```python
from build123d import *

# Parameters (mm, degrees)
CROQUIS1_R              = 4
CROQUIS1_R_2            = 1.25
SALIENTE_EXTRUIR1_DEPTH = 3.5
CROQUIS2_R              = 4
SALIENTE_EXTRUIR2_DEPTH = 150


with BuildPart() as part:
    # Croquis1 → Saliente-Extruir1 (new body)
    # profile 1 of 2: a face of its own
    with BuildSketch(Plane(origin=(0, 0, 0), x_dir=(1, 0, 0), z_dir=(0, 1, 0))):
        with BuildLine():
            Line((17.5, 2.5), (17.5, -2.5))
            ThreePointArc((17.5, -2.5), (16.035533906, -6.035533906), (12.5, -7.5))
            Line((12.5, -7.5), (-12.5, -7.5))
            ThreePointArc((-12.5, -7.5), (-16.035533906, -6.035533906), (-17.5, -2.5))
            Line((-17.5, -2.5), (-17.5, 2.5))
            ThreePointArc((-17.5, 2.5), (-16.035533906, 6.035533906), (-12.5, 7.5))
            Line((-12.5, 7.5), (12.5, 7.5))
            ThreePointArc((12.5, 7.5), (16.035533906, 6.035533906), (17.5, 2.5))
        make_face()
        Circle(CROQUIS1_R, mode=Mode.SUBTRACT)
        with Locations(Location((-13, 0, 0), (0, 0, 270))):
            Circle(CROQUIS1_R_2, mode=Mode.SUBTRACT)
        with Locations(Location((13, 0, 0), (0, 0, 270))):
            Circle(CROQUIS1_R_2, mode=Mode.SUBTRACT)
    # profile 2 of 2: a face of its own
    with BuildSketch(Plane(origin=(0, 0, 0), x_dir=(1, 0, 0), z_dir=(0, 1, 0))):
        Circle(CROQUIS1_R)
    extrude(amount=SALIENTE_EXTRUIR1_DEPTH)

    # Croquis2 → Saliente-Extruir2 (add)
    with BuildSketch(Plane(origin=(0, 3.5, 0), x_dir=(1, 0, 0), z_dir=(0, 1, 0))):
        with Locations(Location((0, 0, 0), (0, 0, 270))):
            Circle(CROQUIS2_R)
    extrude(amount=SALIENTE_EXTRUIR2_DEPTH)


solid = part.part
```
CAD build for the part. Positions are in the model's coordinates, mm. Give positions to 0.01 mm unless a question says otherwise; leave off trailing zeros. Order: outer loops, then holes, each group sorted by start corner. A loop starts at its lowest first (then second) coordinate and runs counter-clockwise, first axis right, second up.
(1) Saw through at C-C, the plane z = -6. Give the cut face in (x, y).
(2) Saw through at D-D, the plane x = 8.5. Give the cut face in (y, z).
(3) Mould opens along X. For faces 1 (the flat face through (-17.5, 2, 0)), 2 (the cylindrical face through (-11.76, 1.73, -0.16)), 3 (the cylindrical face through (-3.905, 77.45, -0.867)), 4 (the flat face through (17.5, 2, 0)) say: released by +X, released by -X, zero draft, split by the parting line, or undercut.
(4) Flat gauge pins, fed straight in: pin 1 (1.5 mm diameter, centred on x = 3.5, y = 94.5, fed in from +Z); pin 2 (1 mm diameter, centred on x = -9.5, z = -4.5, fed in from +Y); pin 3 (3 mm diameter, centred on y = 39.5, z = 0.5, fed in from +X). Where does each tip first touch, or does it go through?
(5) Drill centre lines: L1, parallel to Y at x = 7.5, z = -5.25; L2, parallel to Z at x = 0.5, y = 75.5; L3, parallel to Z at x = 3, y = 15. Where is each one in solid material? Low to high.
(6) Saw through at B-B, the plane y = 86. Give the cut face in (x, z).
(7) Saw through at A-A, the plane x = 0. Give the cut face in (y, z), then the cut area to 3 significant figures.
Results found:
1. outline: (-16.07, 0) - (16.07, 0) - (16.07, 3.5) - (-16.07, 3.5) - close
2. outline: (0, -7.5) - (3.5, -7.5) - (3.5, 7.5) - (0, 7.5) - close
3. face 1: released by -X
3. face 2: undercut
3. face 3: split by the parting line
3. face 4: released by +X
4. pin 1: stops at z = 2.9
4. pin 2: stops at y = 3.5
4. pin 3: stops at x = 4
5. L1: y = 0 to 3.5
5. L2: z = -3.97 to 3.97
5. L3: z = -2.65 to 2.65
6. outline: circle Ø8 at (0, 0)
7. outline: (0, -7.5) - (3.5, -7.5) - (3.5, -4) - (153.5, -4) - (153.5, 4) - (3.5, 4) - (3.5, 7.5) - (0, 7.5) - close
7. area: 1,250 mm2
